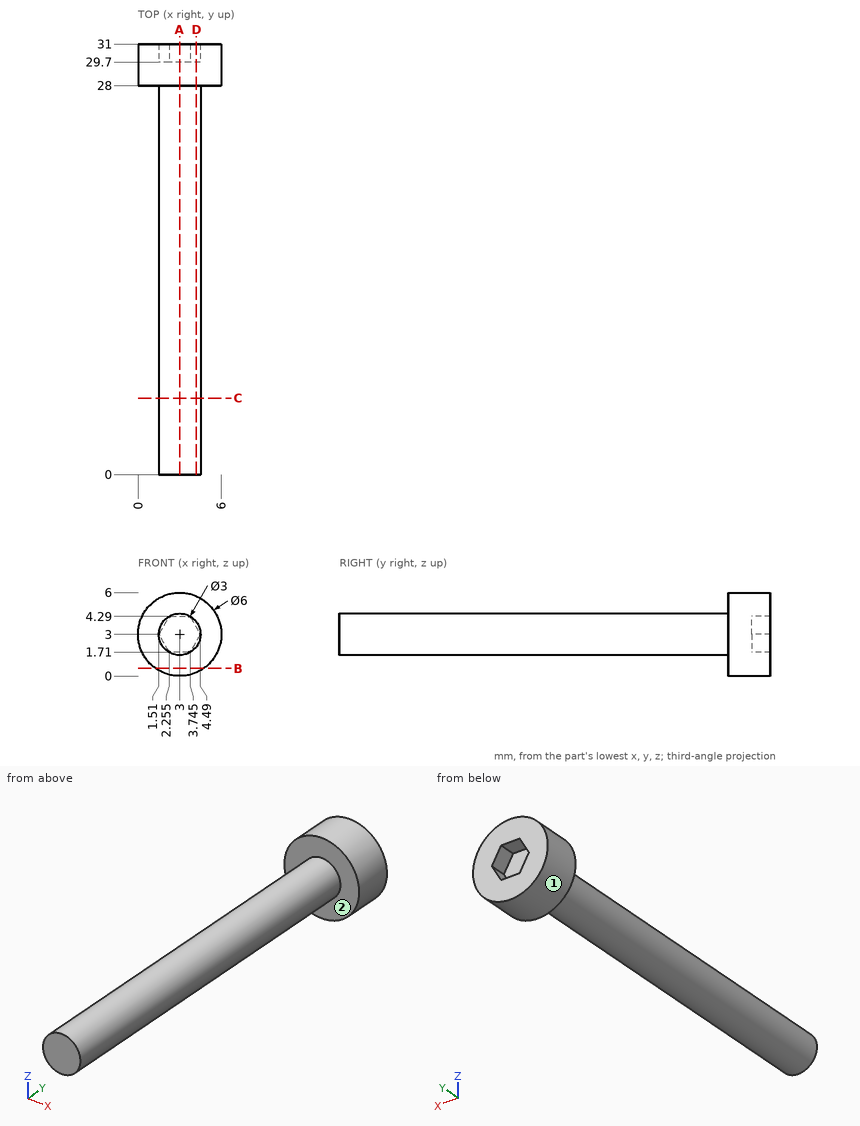
Geometry: see drawing. Coordinates: mm, zero at the bounding-box minimum. A direction names the side the tool comes from. Round coordinates to 2 decimals unless told otherwise and drop trailing zeros. Loops run counter-clockwise (first coordinate to the right, second up) from the corner with the lowest first, then second, coordinate; pieces in that order, holes last. Notation, with made-up numbers: M 20.5,67 L 48.5,67 A23 cw 48.5,80 Z; hole C -6.75,6.5 d5. An arc over 180 degrees is marked long. Use a Markdown table: item, result. Add a question column.
1. Ray query, line 1 along Y through (x, z) = (4.3, 0.85); line 2 along Y through (x, z) = (3.85, 2.15); line 3 along Z through (x, y) = (1.8, 26.5). Return the intervals inside material, ascending. Write a range as [from, to].
2. Cut plane B-B, the plane z = 0.55. Output: boundary loops of the cut face in (x, y).
3. Contact query for flat-ended pins moving along their axis: pin 1 (3 mm diameter, centred on x = 4.5, y = 21, fed in from -Z); pin 2 (3 mm diameter, centred on y = 15.5, z = 3, fed in from +X); pin 3 (2 mm diameter, centred on x = 3, z = 3, fed in from +Y). Output: stop coordinate, or through.
4. Set-up query: the marked faces 1 and 2. Return all of +Z, -Z, +X, -X, +Y, -Y with unobstructed straight access to the full face (end or side cutting, diameter ignored); none if empty.
5. Cut plane D-D, the plane x = 4.2. Output: boundary loops of the cut face in (y, z).
6. Cut plane C-C, the plane y = 5.5. Output: boundary loops of the cut face in (x, z).
7. Cut plane A-A, the plane x = 3. Output: boundary loops of the cut face in (y, z).
Solution:
| question | item | result |
|---|---|---|
| 1 | line 1 | y = [28, 31] |
| 1 | line 2 | y = [0, 29.7] |
| 1 | line 3 | z = [2.1, 3.9] |
| 2 | outline | M 1.27,28 L 4.73,28 L 4.73,31 L 1.27,31 Z |
| 3 | pin 1 | stops at z = 1.5 |
| 3 | pin 2 | stops at x = 4.5 |
| 3 | pin 3 | stops at y = 29.7 |
| 4 | face 1 | +Y, -Y |
| 4 | face 2 | -Y |
| 5 | outline | M 0,2.1 L 28,2.1 L 28,0.25 L 31,0.25 L 31,2.5 L 29.7,2.5 L 29.7,3.5 L 31,3.5 L 31,5.75 L 28,5.75 L 28,3.9 L 0,3.9 Z |
| 6 | outline | C 3,3 d3 |
| 7 | outline | M 0,1.5 L 28,1.5 L 28,0 L 31,0 L 31,1.71 L 29.7,1.71 L 29.7,4.29 L 31,4.29 L 31,6 L 28,6 L 28,4.5 L 0,4.5 Z |
